The listing builds one solid part. Answer for the finished solid, in the listing's coordinates (mm). A direction names the side the tool comes from. Round coordinates to 2 decimals unless told otherwise and drop trailing zeros. Write each loop counter-clockwise with the first axis right and the second up, starting at its lowest first coordinate (ties: lowest second). Pieces come first, ordered by that corner, then holes. Notation, with made-up numbers: (25, -24) - (32, -24) arc R12 ccw to (32, -12) - close; hole circle Ø11 at (-34, 51.25). An arc over 180 degrees is marked (long way). Answer as CSV lines item,"result". Start each with the question number.
Item 1: A cutting plane is placed at A-A on z = 0. Determine the outline of the cut face in (x, y), and give its area (3 significant figures).
Item 2: Flat-ended cylindrical pins translate along their axes: pin 1 (1.5 mm diameter, centred on x = -38.5, y = 1, fed in from -Z); pin 2 (0.9 mm diameter, centred on y = 1, z = 9, fed in from -X); pin 3 (0.9 mm diameter, centred on x = 31, y = 1, fed in from -Z). Find the tip coordinate at first contact, or state that the pin passes through.
Item 3: A cutting plane is placed at C-C on z = 4.25. Determine the outline of the cut face in (x, y), and give its area (4 significant figures).
Item 4: Which of the six approach directions +Z, -Z, +X, -X, +Y, -Y give full straight-line access (tool end or side, diameter ignored) to faces 1 (the flat face through (29.5, 1, -8)), 2 (the flat face through (33.5, 1, 8)), 3 (the flat face through (-37.5, 1, -8))?
Item 5: A cutting plane is placed at D-D on y = 0.95. State how many separate pieces and enclosed holes the cut face has, and give its area (3 significant figures).
Item 6: For a pull along X with two mould halves and no side action, classify faces 4 (the cylindrical face through (-33.11, 1.48, -0.16)), 5 (the flat face through (-12, 1, 10)), 6 (the flat face through (-40.5, 1, -4)) as pulls with the +X half, pulls with the -X half, needs draft (parallel to the pull), parting line crosses it, or undercut.
Item 7: Straight lines are drawn through the part: line 1 along X through (y, z) = (1.4, 0); line 2 along Z through (x, y) = (11.5, 1); line 3 along X through (y, z) = (1.9, 3). For each, find the intervals that lie inside material, in ascending order. Write a range as [from, to].
Item 8: A cutting plane is placed at B-B on x = -6.15. Determine the outline of the cut face in (y, z), and give its area (3 significant figures).
```python
from build123d import *

# Parameters (mm, degrees)
CROQUIS1_R              = 1.25
CROQUIS1_W              = 22.5
CROQUIS1_H              = 12.5
CROQUIS1_R_2            = 3.6
CROQUIS1_W_2            = 3
CROQUIS1_H_2            = 4
SALIENTE_EXTRUIR1_DEPTH = 3


with BuildPart() as part:
    # Croquis1 → Saliente-Extruir1 (new body)
    # profile 1 of 3: a face of its own
    with BuildSketch(Plane(origin=(0, 0, 0), x_dir=(1, 0, 0), z_dir=(0, 1, 0))):
        Polygon((-37.5, -6), (-37.5, -10), (13.5, -10), (13.5, -7), (17.5, -7), (17.5, -10), (21.5, -10), (21.5, -7), (25.5, -7), (25.5, -10), (29.5, -10), (29.5, -7), (33.5, -7), (33.5, -10), (37.5, -10), (37.5, 10), (33.5, 10), (33.5, 7), (29.5, 7), (29.5, 10), (25.5, 10), (25.5, 7), (21.5, 7), (21.5, 10), (17.5, 10), (17.5, 7), (13.5, 7), (13.5, 10), (-37.5, 10), (-37.5, 6), (-37.5, 2), (-37.5, -2), align=None)
        with Locations(Location((-34.35, 0, 0), (0, 0, 270))):
            Circle(CROQUIS1_R, mode=Mode.SUBTRACT)
        with Locations((-20.25, 0)):
            Rectangle(CROQUIS1_W, CROQUIS1_H, mode=Mode.SUBTRACT)
        with Locations(Location((-6.15, 0, 0), (0, 0, 270))):
            Circle(CROQUIS1_R, mode=Mode.SUBTRACT)
        with Locations(Location((14.5, 0, 0), (0, 0, 270))):
            Circle(CROQUIS1_R_2, mode=Mode.SUBTRACT)
    # profile 2 of 3: a face of its own
    with BuildSketch(Plane(origin=(0, 0, 0), x_dir=(1, 0, 0), z_dir=(0, 1, 0))):
        with Locations((-39, -4)):
            Rectangle(CROQUIS1_W_2, CROQUIS1_H_2)
    # profile 3 of 3: a face of its own
    with BuildSketch(Plane(origin=(0, 0, 0), x_dir=(1, 0, 0), z_dir=(0, 1, 0))):
        with Locations((-39, 4)):
            Rectangle(CROQUIS1_W_2, CROQUIS1_H_2)
    extrude(amount=SALIENTE_EXTRUIR1_DEPTH)


solid = part.part
```
Geometry says:
1,outline,"(-37.5, 0) - (-35.6, 0) - (-35.6, 3) - (-37.5, 3) - close; (-33.1, 0) - (-31.5, 0) - (-31.5, 3) - (-33.1, 3) - close; (-9, 0) - (-7.4, 0) - (-7.4, 3) - (-9, 3) - close; (-4.9, 0) - (10.9, 0) - (10.9, 3) - (-4.9, 3) - close; (18.1, 0) - (37.5, 0) - (37.5, 3) - (18.1, 3) - close"
1,area,"121 mm^2"
2,pin 1,"stops at z = -6"
2,pin 2,"stops at x = -37.5"
2,pin 3,"stops at z = -7"
3,outline,"(-40.5, 0) - (-31.5, 0) - (-31.5, 3) - (-40.5, 3) - close; (-9, 0) - (37.5, 0) - (37.5, 3) - (-9, 3) - close"
3,area,"166.5 mm^2"
4,face 1,"-Z, +Y, -Y"
4,face 2,"+Z, +Y, -Y"
4,face 3,"-Z, -X, +Y, -Y"
5,separate pieces,"1"
5,enclosed holes,"4"
5,area,"1,120 mm^2"
6,face 4,"undercut"
6,face 5,"needs draft"
6,face 6,"pulls with the -X half"
7,line 1,"x = [-37.5, -35.6], [-33.1, -31.5], [-9, -7.4], [-4.9, 10.9], [18.1, 37.5]"
7,line 2,"z = [-10, -1.99], [1.99, 10]"
7,line 3,"x = [-40.5, -31.5], [-9, 12.51], [16.49, 37.5]"
8,outline,"(0, -10) - (3, -10) - (3, -1.25) - (0, -1.25) - close; (0, 1.25) - (3, 1.25) - (3, 10) - (0, 10) - close"
8,area,"52.5 mm^2"
